Build history of the part. All positions in model axes, mm. Give positions to 0.01 mm unless a question says otherwise; leave off trailing zeros. Loops run counter-clockwise (first coordinate to the right, second up) from the corner with the lowest first, then second, coordinate; pieces in that order, holes last. Notation, with made-up numbers: M -32.5,-10 L 3.5,-10 A11 cw 3.5,-3 Z; hole C -17.5,41 d8. An arc over 180 degrees is marked long. Answer as a JSON object with one key per item and string values. Group by question number.
1. Drill centre lines: line 1 along Z through (x, y) = (5.5, -1.25) (1 decimal); line 2 along Y through (x, z) = (-0.25, 992); line 3 along X through (y, z) = (0, 679.5). Where is each one in solid material? Low to high. Write a range as [from, to].
2. Drop flat-ended pins along their axis: pin 1 Ø2 at (x, z) = (3, 225.5) entering from -Y; pin 2 Ø3 at (x, z) = (-5, 694.5) entering from -Y; pin 3 Ø1 at (x, y) = (3.5, 4) entering from -Z; pin 4 Ø2 at (x, z) = (-4.5, 871) entering from +Y. Give the stop position or say it passes through.
3. Slice it at A-A (x = 0). List the corners of the cut face in (y, z) (1 decimal), then the cut area to 3 significant figures.
4. Slice it at C-C (z = 192). List the corners of the cut face in (x, y).
from build123d import *

# Parameters (mm, degrees)
SKETCH1_R           = 5
BOSS_EXTRUDE1_DEPTH = 1069.975
SKETCH2_W           = 15
SKETCH2_H           = 15
BOSS_EXTRUDE2_DEPTH = 117.475
SKETCH3_W           = 15
SKETCH3_H           = 15
BOSS_EXTRUDE3_DEPTH = 20.6375


with BuildPart() as part:
    # Sketch1 → Boss-Extrude1 (new body)
    with BuildSketch(Plane.XY):
        Circle(SKETCH1_R)
    extrude(amount=BOSS_EXTRUDE1_DEPTH)

    # Sketch2 → Boss-Extrude2 (add)
    with BuildSketch(Plane.XY):
        Rectangle(SKETCH2_W, SKETCH2_H)
    extrude(amount=BOSS_EXTRUDE2_DEPTH)

    # Sketch3 → Boss-Extrude3 (add)
    with BuildSketch(Plane.XY.offset(1069.975)):
        Rectangle(SKETCH3_W, SKETCH3_H)
    extrude(amount=-BOSS_EXTRUDE3_DEPTH)


solid = part.part
Established:
{
 "1": {"line 1": "z = [0, 117.5], [1049.3, 1070]", "line 2": "y = [-4.99, 4.99]", "line 3": "x = [-5, 5]"},
 "2": {"pin 1": "stops at y = -4.58", "pin 2": "stops at y = -3.57", "pin 3": "stops at z = 0", "pin 4": "stops at y = 3.57"},
 "3": {"outline": "M -7.5,0 L 7.5,0 L 7.5,117.5 L 5,117.5 L 5,1049.3 L 7.5,1049.3 L 7.5,1070 L -7.5,1070 L -7.5,1049.3 L -5,1049.3 L -5,117.5 L -7.5,117.5 Z", "area": "11,400 mm^2"},
 "4": {"outline": "C 0,0 d10"}
}
